Geometry: final body of the model. Coordinates: model frame, mm. A direction names the side the tool comes from. Give positions to 0.01 mm unless a question says otherwise; leave off trailing zeros. Write each loop counter-clockwise with the first axis right and the second up, starting at its lowest first coordinate (ties: lowest second). Pieces come first, ordered by that corner, then holes. Notation, with made-up numbers: M 50,71.25 L 55,71.25 A25 cw 55,85.25 Z; hole C -26,7.25 d11. An arc over 180 degrees is marked long. Answer as a JSON object with one key per item and string values.
from build123d import *

# Parameters (mm, degrees)
SKETCH1_W           = 45
SKETCH1_H           = 40
BOSS_EXTRUDE1_DEPTH = 2
SKETCH2_W           = 2
SKETCH2_H           = 42.8
BOSS_EXTRUDE2_DEPTH = 45
FILLET1_R           = 1
SKETCH3_W           = 2
SKETCH3_H           = 13
CUT_EXTRUDE1_DEPTH  = 11
SKETCH4_W           = 8
SKETCH4_H           = 20
CUT_EXTRUDE2_DEPTH  = 11


with BuildPart() as part:
    # Sketch1 → Boss-Extrude1 (new, symmetric)
    with BuildSketch(Plane.XY):
        with BuildLine():
            Line((-22.555173768, -23.917239348), (22.044826232, -23.917239348))
            ThreePointArc((22.044826232, -23.917239348), (24.166146575, -23.038559691), (25.044826232, -20.917239348))
            Line((25.044826232, -20.917239348), (25.044826232, 21.682760652))
            ThreePointArc((25.044826232, 21.682760652), (24.166146575, 23.804080996), (22.044826232, 24.682760652))
            Line((22.044826232, 24.682760652), (-22.555173768, 24.682760652))
            ThreePointArc((-22.555173768, 24.682760652), (-24.676494112, 23.804080996), (-25.555173768, 21.682760652))
            Line((-25.555173768, 21.682760652), (-25.555173768, -20.917239348))
            ThreePointArc((-25.555173768, -20.917239348), (-24.676494112, -23.038559691), (-22.555173768, -23.917239348))
        make_face()
        with Locations((-0.255173768, 1.882760652)):
            Rectangle(SKETCH1_W, SKETCH1_H, mode=Mode.SUBTRACT)
    extrude(amount=BOSS_EXTRUDE1_DEPTH, both=True)

    # Sketch2 → Boss-Extrude2 (add)
    with BuildSketch(Plane(origin=(-22.755173768, 0, 0), x_dir=(0, 0, -1), z_dir=(1, 0, 0))):
        with Locations((-1, 0.482760652)):
            Rectangle(SKETCH2_W, SKETCH2_H)
    extrude(amount=BOSS_EXTRUDE2_DEPTH)

    # Fillet1
    fillet1_edges = [part.edges().sort_by_distance(p)[0] for p in [
        (22.244826232, 21.882760652, -1),
        (-22.755173768, 21.882760652, -1),
        (22.244826232, -18.117239348, -1),
        (-22.755173768, -18.117239348, -1),
        (-0.255173768, -18.117239348, 0),
        (-0.255173768, 21.882760652, 0),
        (-22.755173768, 1.882760652, 0),
        (22.244826232, 1.882760652, 0),
    ]]
    fillet(fillet1_edges, radius=FILLET1_R)

    # Sketch3 → Cut-Extrude1 (cut)
    with BuildSketch(Plane.ZY.offset(25.555173768)):
        with Locations((-1, -0.417239348)):
            Rectangle(SKETCH3_W, SKETCH3_H)
    extrude(amount=-CUT_EXTRUDE1_DEPTH, mode=Mode.SUBTRACT)

    # Sketch4 → Cut-Extrude2 (cut)
    with BuildSketch(Plane.XY.offset(2)):
        with Locations((19.044826232, 1.082760652)):
            Rectangle(SKETCH4_W, SKETCH4_H)
    extrude(amount=-CUT_EXTRUDE2_DEPTH, mode=Mode.SUBTRACT)


solid = part.part
1) Cut plane A-A on x = 19.5. Return loops of the section in (y, z), and give its area (3 significant figures).
Geometry check:
{"outline": "M -23.92,-2 L -18.12,-2 L -18.12,-1 A1 cw -17.12,0 L -8.92,0 L -8.92,2 L -23.92,2 Z; M 11.08,0 L 20.88,0 A1 cw 21.88,-1 L 21.88,-2 L 24.68,-2 L 24.68,2 L 11.08,2 Z", "area": "74.8 mm2"}
2) Line query: line 1 (X direction, y = -6.5, z = 0.6); line 2 (X direction, y = -11, z = -1.4); line 3 (Y direction, x = -8.5, z = -1.8). Output: solid intervals per line, ascending. Write a range as from..to.
Geometry check:
{"line 1": "x = -25.56..15.04, 23.04..25.04", "line 2": "x = -25.56..-22.76, 22.24..25.04", "line 3": "y = -23.92..-18.12, 21.88..24.68"}
3) Set-up query: faces 1 (the flat face through (25.045, 0, 0)), 2 (the flat face through (-24, 6.083, -1)), 3 (the flat face through (15.045, 1, 1)), 4 (the flat face through (-2, 2, 0)). Return all of +Z, -Z, +X, -X, +Y, -Y with unobstructed straight access to the full face (end or side cutting, diameter ignored); none if empty.
Geometry check:
{"face 1": "+Z, -Z, +X, +Y, -Y", "face 2": "-Z, -X", "face 3": "+Z, -Z", "face 4": "-Z"}
4) Cut plane B-B on y = -1.5. Return loops of the section in (x, z).
Geometry check:
{"outline": "M -25.56,0 L 15.04,0 L 15.04,2 L -25.56,2 Z; M 23.04,-2 L 25.04,-2 L 25.04,2 L 23.04,2 Z"}
5) Pull-direction query (Y, two-part tool) for faces 5 (the flat face through (19, -8.917, 1)), 6 (the flat face through (0, -19, -2)), 7 (the flat face through (23.045, 1, 0)), 8 (the flat face through (0, 24.683, 0)); classes: pulls with the +Y half, pulls with the -Y half, needs draft (parallel to the pull), parting line crosses it, or undercut.
Geometry check:
{"face 5": "undercut", "face 6": "needs draft", "face 7": "undercut", "face 8": "pulls with the +Y half"}
6) Contact query for flat-ended pins moving along their axis: P1, Ø1, axis at x = 10.5, y = 2.5, coming from the -Z side; P2, Ø2, axis at x = -24.5, z = -0.5, coming from the -Y side; P3, Ø1, axis at x = -24, z = -1, coming from the +Y side. Output: stop coordinate, or through.
Geometry check:
{"P1": "stops at z = 0", "P2": "stops at y = -23.76", "P3": "stops at y = 24.53"}
7) Cut plane D-D on x = -6. Return loops of the section in (y, z).
Geometry check:
{"outline": "M -23.92,-2 L -18.12,-2 L -18.12,-1 A1 cw -17.12,0 L 20.88,0 A1 cw 21.88,-1 L 21.88,-2 L 24.68,-2 L 24.68,2 L -23.92,2 Z"}
8) Cut plane C-C on z = 1.05. Return loops of the section in (x, y).
Geometry check:
{"outline": "M -25.56,-20.92 A3 ccw -22.56,-23.92 L 22.04,-23.92 A3 ccw 25.04,-20.92 L 25.04,21.68 A3 ccw 22.04,24.68 L -22.56,24.68 A3 ccw -25.56,21.68 Z; hole M 15.04,-8.92 L 23.04,-8.92 L 23.04,11.08 L 15.04,11.08 Z"}
